Verification items for the finished model (mm, model axes). A direction names the side the tool comes from. Coordinates: 2 decimals unless noted, no trailing zeros. Write each loop counter-clockwise with the first axis right and the second up, starting at its lowest first coordinate (ties: lowest second). Pieces come first, ordered by that corner, then holes. Notation, with made-up numbers: (86, -12.75) - (105, -12.75) arc R15 ccw to (105, 10.25) - close; hole circle Ø8 at (1.5, 16.25). An arc over 180 degrees is marked (long way). Use one line per item in the form item = value. Start each with the question number.
(1) Material ranges on line 1 (X direction, y = 3.5, z = -13.5); line 2 (Z direction, x = 0, y = 14.5), recorded low to high. Write a range as [from, to].
(2) Mould release check, pull along Z, two halves, no side actions. Record for faces 1 (the flat face through (-17.6, 9.9, -5)), 2 (the flat face through (0, 10, -10)), 3 (the flat face through (5, 10, -17)): released by +Z, released by -Z, zero draft, split by the parting line, or undercut.
(3) Tool access check on faces 4 (the flat face through (10, 10, 17)), 5 (the cylindrical face through (9.1, 19.14, -0.07)), 6 (the flat face through (-17, 10, 10)), 7 (the flat face through (0, 10, 3.1)). Record the directions out of +Z, -Z, +X, -X, +Y, -Y that give a thin tool (end or side, any length) a straight path to the whole face; none if there is none.
(4) Sectioned sample at C-C (x = 19.5). Record the cut outline in (y, z).
(5) Sectioned sample at B-B (z = -3). Record the cut outline in (x, y), and give its area (3 significant figures).
(6) Sectioned sample at A-A (x = 0). Record the cut outline in (y, z).
(7) Gauge pin test, flat ends, axial feed: pin 1 Ø4 at (x, z) = (-17.5, 1.5) entering from -Y; pin 2 Ø1.5 at (y, z) = (2.5, -14.5) entering from -X; pin 3 Ø9 at (y, z) = (10.5, 16.5) entering from +X; pin 4 Ø8 at (x, y) = (0, 10) entering from +Z. Record the tip position at first contact, or that the pin passes through.
from build123d import *

# Parameters (mm, degrees)
SKETCH1_W           = 20
SKETCH1_H           = 20
SKETCH1_W_2         = 18
SKETCH1_H_2         = 5
SKETCH1_W_3         = 5
SKETCH1_H_3         = 18
BOSS_EXTRUDE1_DEPTH = 20
FILLET1_R           = 10
SKETCH2_R           = 2.6
CUT_EXTRUDE1_DEPTH  = 20
CIRPATTERN1_COUNT   = 4
FILLET2_R           = 3


with BuildPart() as part:
    # Sketch1 → Boss-Extrude1 (new body)
    # profile 1 of 9: a face of its own
    with BuildSketch(Plane(origin=(0, 0, 0), x_dir=(1, 0, 0), z_dir=(0, 1, 0))):
        Rectangle(SKETCH1_W, SKETCH1_H)
        with BuildLine():
            ThreePointArc((2.606242506, -3.1), (0, 4.05), (-2.606242506, -3.1))
            Line((-2.606242506, -3.1), (2.606242506, -3.1))
        make_face(mode=Mode.SUBTRACT)
    # profile 2 of 9: a face of its own
    with BuildSketch(Plane(origin=(0, 0, 0), x_dir=(1, 0, 0), z_dir=(0, 1, 0))):
        with Locations((-19, -7.5)):
            Rectangle(SKETCH1_W_2, SKETCH1_H_2)
    # profile 3 of 9: a face of its own
    with BuildSketch(Plane(origin=(0, 0, 0), x_dir=(1, 0, 0), z_dir=(0, 1, 0))):
        with Locations((-19, 7.5)):
            Rectangle(SKETCH1_W_2, SKETCH1_H_2)
    # profile 4 of 9: a face of its own
    with BuildSketch(Plane(origin=(0, 0, 0), x_dir=(1, 0, 0), z_dir=(0, 1, 0))):
        with Locations((-7.5, 19)):
            Rectangle(SKETCH1_W_3, SKETCH1_H_3)
    # profile 5 of 9: a face of its own
    with BuildSketch(Plane(origin=(0, 0, 0), x_dir=(1, 0, 0), z_dir=(0, 1, 0))):
        with Locations((7.5, 19)):
            Rectangle(SKETCH1_W_3, SKETCH1_H_3)
    # profile 6 of 9: a face of its own
    with BuildSketch(Plane(origin=(0, 0, 0), x_dir=(1, 0, 0), z_dir=(0, 1, 0))):
        with Locations((19, 7.5)):
            Rectangle(SKETCH1_W_2, SKETCH1_H_2)
    # profile 7 of 9: a face of its own
    with BuildSketch(Plane(origin=(0, 0, 0), x_dir=(1, 0, 0), z_dir=(0, 1, 0))):
        with Locations((19, -7.5)):
            Rectangle(SKETCH1_W_2, SKETCH1_H_2)
    # profile 8 of 9: a face of its own
    with BuildSketch(Plane(origin=(0, 0, 0), x_dir=(1, 0, 0), z_dir=(0, 1, 0))):
        with Locations((7.5, -19)):
            Rectangle(SKETCH1_W_3, SKETCH1_H_3)
    # profile 9 of 9: a face of its own
    with BuildSketch(Plane(origin=(0, 0, 0), x_dir=(1, 0, 0), z_dir=(0, 1, 0))):
        with Locations((-7.5, -19)):
            Rectangle(SKETCH1_W_3, SKETCH1_H_3)
    extrude(amount=BOSS_EXTRUDE1_DEPTH)

    # Fillet1
    fillet1_edges = [part.edges().sort_by_distance(p)[0] for p in [
        (-28, 0, 7.5),
        (-28, 20, 7.5),
        (-28, 0, -7.5),
        (-28, 20, -7.5),
        (-7.5, 0, -28),
        (-7.5, 20, -28),
        (7.5, 0, -28),
        (7.5, 20, -28),
        (28, 0, -7.5),
        (28, 20, -7.5),
        (28, 0, 7.5),
        (28, 20, 7.5),
        (7.5, 0, 28),
        (7.5, 20, 28),
        (-7.5, 0, 28),
        (-7.5, 20, 28),
    ]]
    fillet(fillet1_edges, radius=FILLET1_R - 0.0001)  # a hair under: the kernel refuses the full size

    # Sketch2 → Cut-Extrude1 (cut)
    with BuildSketch(Plane.XY.offset(10)):
        with Locations((-20.5, 10)):
            Circle(SKETCH2_R)
    cut_extrude1 = extrude(amount=-CUT_EXTRUDE1_DEPTH, mode=Mode.SUBTRACT)

    # CirPattern1: Cut-Extrude1 ×4 about axis
    cirpattern1_axis = Axis((0, 21, 0), (0, -1, 0))
    for i in range(1, CIRPATTERN1_COUNT):
        add(cut_extrude1.rotate(cirpattern1_axis, i * 360 / CIRPATTERN1_COUNT), mode=Mode.SUBTRACT)

    # Fillet2
    fillet2_edges = [part.edges().sort_by_distance(p)[0] for p in [
        (-10, 20, 0),
        (0, 20, 10),
        (-10, 0, 0),
        (0, 0, -10),
        (10, 0, 0),
        (0, 0, 10),
        (10, 20, 0),
        (0, 20, -10),
    ]]
    fillet(fillet2_edges, radius=FILLET2_R)


solid = part.part
Answers below:
q1.line_1 = [-10, -5], [5, 10]
q1.line_2 = [-10, -4.05], [3.1, 10]
q2.face_1 = undercut
q2.face_2 = released by -Z
q2.face_3 = zero draft
q3.face_4 = +Z, +X, +Y, -Y
q3.face_5 = +X, +Y
q3.face_6 = +Z, -X, +Y, -Y
q3.face_7 = +Y, -Y
q4.outline = (0.11, -10) - (7.6, -10) - (7.6, -5) - (0.11, -5) - close; (0.11, 5) - (7.6, 5) - (7.6, 10) - (0.11, 10) - close; (12.4, -10) - (19.89, -10) - (19.89, -5) - (12.4, -5) - close; (12.4, 5) - (19.89, 5) - (19.89, 10) - (12.4, 10) - close
q5.outline = (-10, 3) arc R3 ccw to (-7, 0) - (-2.72, 0) - (-2.72, 20) - (-7, 20) arc R3 ccw to (-10, 17) - close; (2.72, 0) - (7, 0) arc R3 ccw to (10, 3) - (10, 17) arc R3 ccw to (7, 20) - (2.72, 20) - close
q5.area = 283 mm2
q6.outline = (0, -7) arc R3 ccw to (3, -10) - (17, -10) arc R3 ccw to (20, -7) - (20, -4.05) - (0, -4.05) - close; (0, 3.1) - (20, 3.1) - (20, 7) arc R3 ccw to (17, 10) - (3, 10) arc R3 ccw to (0, 7) - close
q7.pin_1 = through
q7.pin_2 = -10
q7.pin_3 = 10
q7.pin_4 = 10
